```python
from build123d import *


with BuildPart() as part:
    # Sketch2 → Revolve1 (revolve)
    with BuildSketch(Plane.XY, mode=Mode.PRIVATE) as revolve1_sk:
        with BuildLine():
            Line((0.5334, 11.2268), (0.5334, 9.4742))
            Line((0.5334, 9.4742), (0.7493, 9.4742))
            Line((0.7493, 9.4742), (0.7493, 4.9022))
            Line((0.7493, 4.9022), (0.9144, 4.9022))
            Line((0.9144, 4.9022), (0.9144, 3.683))
            Line((0.9144, 3.683), (0.9906, 3.683))
            Line((0.9906, 3.683), (0.9906, 3.048))
            Line((0.9906, 3.048), (0.8255, 3.048))
            Line((0.8255, 3.048), (0.8255, 0))
            Line((0.8255, 0), (0, 0))
            Line((0, 0), (0, 11.7602))
            ThreePointArc((0, 11.7602), (0.377170757, 11.603970757), (0.5334, 11.2268))
        make_face()
    revolve(revolve1_sk.sketch.rotate(Axis((0, 0, 0), (0, -1, 0)), 90), axis=Axis((0, 0, 0), (0, -1, 0)))


solid = part.part
```
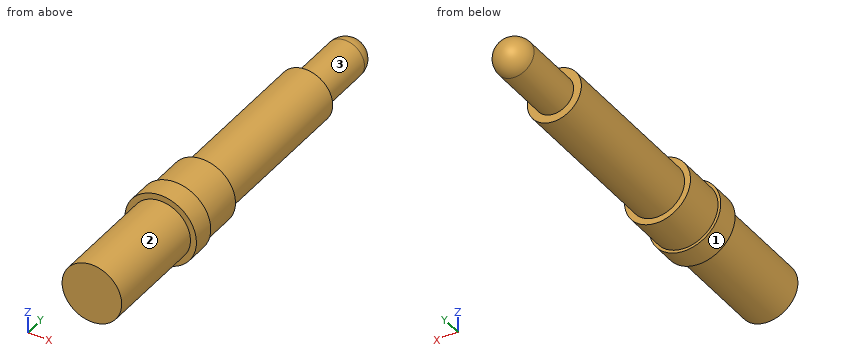
Here's how the part is built. I have some questions about the finished solid (model axes, mm). Face numbers are marked on the shaded views. A direction names the side the tool comes from. Give positions to 0.01 mm unless a question says otherwise; leave off trailing zeros. Write each loop counter-clockwise with the first axis right and the second up, starting at its lowest first coordinate (ties: lowest second). Pieces come first, ordered by that corner, then holes. Notation, with made-up numbers: (-36.5, 50.25) -> (-2.5, 50.25) arc R23 cw to (-2.5, 75.25) -> close; hole circle Ø10 at (48.25, -32). An arc over 180 degrees is marked (long way). Write each question's results on one line, items separated by ' | '.
Item 1: Suppose I cut it at C-C on y = 7.5. Write out the boundary of the cut face in (x, z).
Output:
outline: circle Ø1.5 at (0, 0)
Item 2: Suppose I cut it at A-A on x = 0. Write out the boundary of the cut face in (y, z), plus the area to 3 significant figures.
Output:
outline: (0, -0.83) -> (3.05, -0.83) -> (3.05, -0.99) -> (3.68, -0.99) -> (3.68, -0.91) -> (4.9, -0.91) -> (4.9, -0.75) -> (9.47, -0.75) -> (9.47, -0.53) -> (11.23, -0.53) arc R0.53 ccw to (11.23, 0.53) -> (9.47, 0.53) -> (9.47, 0.75) -> (4.9, 0.75) -> (4.9, 0.91) -> (3.68, 0.91) -> (3.68, 0.99) -> (3.05, 0.99) -> (3.05, 0.83) -> (0, 0.83) -> close | area: 17.7 mm^2
Item 3: On a 3-axis mill with a long thin cutter (end or side, diameter ignored), from which of +Z, -Z, +X, -X, +Y, -Y can I reach the whole of each face in a straight line? I mean the marked faces 1, 2 and 3. Say none if no direction works.
Output:
face 1: +Y, -Y | face 2: -Y | face 3: +Y
Item 4: Suppose I cut it at B-B on z = 0. Write out the boundary of the cut face in (x, y).
Output:
outline: (-0.99, 3.05) -> (-0.83, 3.05) -> (-0.83, 0) -> (0.83, 0) -> (0.83, 3.05) -> (0.99, 3.05) -> (0.99, 3.68) -> (0.91, 3.68) -> (0.91, 4.9) -> (0.75, 4.9) -> (0.75, 9.47) -> (0.53, 9.47) -> (0.53, 11.23) arc R0.53 ccw to (-0.53, 11.23) -> (-0.53, 9.47) -> (-0.75, 9.47) -> (-0.75, 4.9) -> (-0.91, 4.9) -> (-0.91, 3.68) -> (-0.99, 3.68) -> close
Item 5: If I drill on L1, parallel to Y at x = -0.65, z = 0.2; L2, parallel to Y at x = 0.65, z = 0.6; L3, parallel to Z at x = -0.15, y = 3.5, over which ranges is the centre line in solid material (lowest first)?
Output:
L1: y = 0 to 9.47 | L2: y = 3.05 to 4.9 | L3: z = -0.98 to 0.98
Item 6: For pin 1 Ø0.7 at (x, z) = (0, -0.5) entering from +Y; pin 2 Ø1 at (x, z) = (0, 0.5) entering from -Y, each with a flat end and sliding along its axis, tell me the tip position at first contact or that it passes through.
Output:
pin 1: stops at y = 11.74 | pin 2: stops at y = 0
